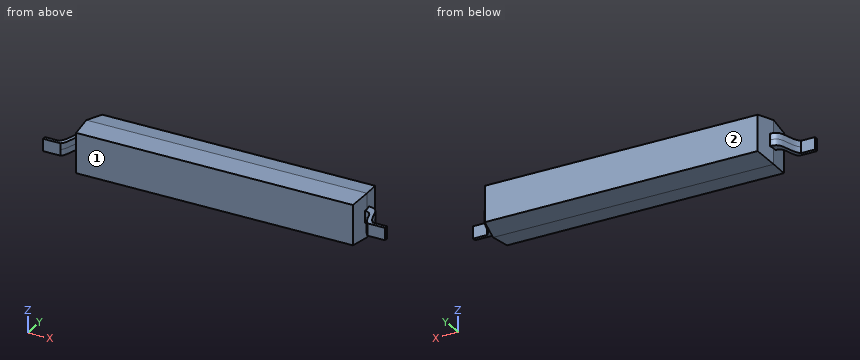
```python
from build123d import *

# Parameters (mm, degrees)
SKETCH_2_W                = 16
SKETCH_2_H                = 2.5
EXTRUDE_1_DEPTH           = 1.25
EXTRUDE_1_TAPER           = 10
EXTRUDE_1_OTHER_WAY_DEPTH = 1.25
EXTRUDE_1_OTHER_WAY_TAPER = 5
EXTRUDE_2_DEPTH           = 0.35


with BuildPart() as part:
    # Эскиз2 → Бобышка-Вытянуть1 (new body)
    with BuildSketch(Plane(origin=(0, 0, 0), x_dir=(1, 0, 0), z_dir=(0, 1, 0))):
        Rectangle(SKETCH_2_W, SKETCH_2_H)
    extrude(amount=EXTRUDE_1_DEPTH, taper=EXTRUDE_1_TAPER)

    # Эскиз2 → Бобышка-Вытянуть1 other way (add)
    with BuildSketch(Plane(origin=(0, 0, 0), x_dir=(1, 0, 0), z_dir=(0, 1, 0))):
        Rectangle(SKETCH_2_W, SKETCH_2_H)
    extrude(amount=-EXTRUDE_1_OTHER_WAY_DEPTH, taper=EXTRUDE_1_OTHER_WAY_TAPER)

    # Эскиз3 → Бобышка-Вытянуть2 (add, symmetric)
    with BuildSketch(Plane.XY):
        with BuildLine():
            Line((-8.94, -1.1), (-9.75, -1.1))
            Line((-9.75, -1.1), (-9.75, -1.3))
            Line((-9.75, -1.3), (-8.75, -1.3))
            add(Edge.make_bspline(
                [(-8.75, -1.3), (-8.598827161, -1.168647342), (-8.520234343, -0.919812082), (-8.367054145, -0.306395683), (-8.139808897, -0.193393407), (-7.92698735, -0.193393407)],
                knots=[0, 0, 0, 0, 0.417832957, 0.685176508, 1, 1, 1, 1], degree=3))
            Line((-7.92698735, -0.193393407), (-7.373029008, -0.193393407))
            Line((-7.373029008, -0.193393407), (-7.373029008, 0.306606593))
            Line((-7.373029008, 0.306606593), (-7.889795637, 0.306606593))
            add(Edge.make_bspline(
                [(-8.94, -1.1), (-8.782709202, -0.94416904), (-8.601427611, -0.451853298), (-8.504762441, 0.074209929), (-8.230463242, 0.306606593), (-7.889795637, 0.306606593)],
                knots=[0, 0, 0, 0, 0.318526042, 0.678515107, 1, 1, 1, 1], degree=3))
        make_face()
    extrude_2 = extrude(amount=EXTRUDE_2_DEPTH, both=True)

    # Зеркальное отражение1: Бобышка-Вытянуть2 across plane
    add(extrude_2.mirror(Plane(origin=(0, 0, 0), x_dir=(0, 0, 1), z_dir=(1, 0, 0))))


solid = part.part
```
Check sheet for the modelled part. Datum: model origin and axes. Units: mm. Face numbers are marked on the shaded views. Coordinates: 2 decimals unless noted, no trailing zeros. Use one line per item in the form item = value.
Item 1: Material ranges on L1, parallel to Y at x = -4.25, z = 0.5; L2, parallel to X at y = 0.1, z = 0.9; L3, parallel to X at y = 0.3, z = 1, recorded low to high. Write a range as from..to.
Answer below:
L1 = -1.25..1.25
L2 = -7.98..7.98
L3 = -7.95..7.95
Item 2: Release check for a two-part mould opening along X. For the marked faces 1 and 2 record: pulls with the +X half, pulls with the -X half, needs draft (parallel to the pull), parting line crosses it, or undercut.
Answer below:
face_1 = undercut
face_2 = needs draft
Item 3: Gauge pin test, flat ends, axial feed: pin 1 Ø0.8 at (x, y) = (-9, -0.5) entering from -Z; pin 2 Ø1.1 at (x, z) = (-3.5, 0.5) entering from -Y; pin 3 Ø1 at (y, z) = (0.5, -1) entering from +X; pin 4 Ø0.5 at (x, y) = (9.5, 0) entering from +Z. Record the tip position at first contact, or that the pin passes through.
Answer below:
pin_1 = -0.35
pin_2 = -1.25
pin_3 = 8
pin_4 = through
Item 4: Sectioned sample at A-A, the plane y = -0.9. State how many separate pieces and enclosed holes the cut face has, and give its area (3 significant figures).
Answer below:
separate_pieces = 3
enclosed_holes = 0
area = 37.5 mm^2
